Design review of the part shown in the three views and the two pictorial views. Dimensions are in mm from the part's minimum x, y and z. A direction names the side the tool comes from. Coordinates: 2 decimals unless noted, no trailing zeros. Order: outer loops, then holes, each group sorted by start corner. A loop starts at its lowest first (then second) coordinate and runs counter-clockwise, first axis right, second up. Notation, with made-up numbers: M 13,84 L 36,84 A10 ccw 36,95 Z; hole C -16.75,42 d11. An arc over 180 degrees is marked long. Use CSV: the item, a comma, the result in double quotes.
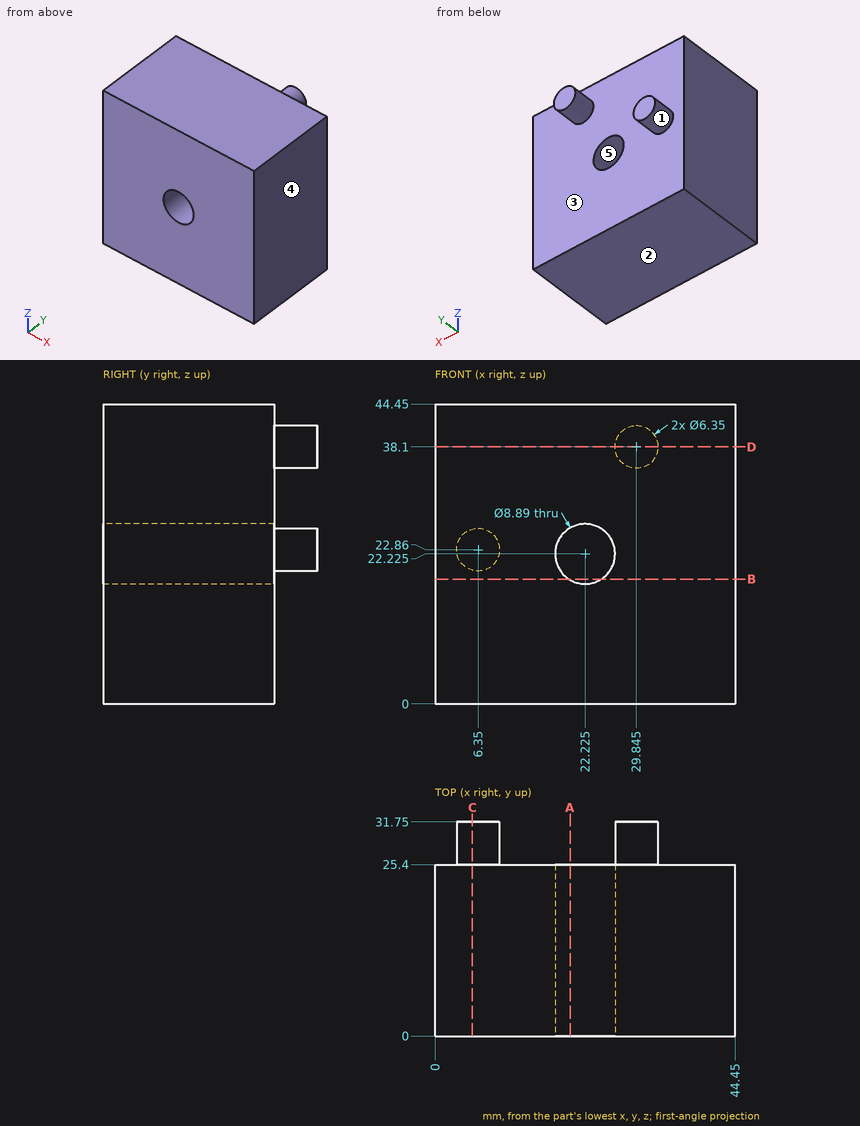
(1) For the marked faces 1 and 2, list the 3-axis set-ups (+Z, -Z, +X, -X, +Y, -Y) from which the entire face can be reached by the end or side of a thin tool; tool diameter is ignored.
The answers:
face 1,"+Y"
face 2,"-Z, +X, -X, +Y, -Y"
(2) The part is to be moulded in two halves that separate along X. For the marked faces 3, 4 and 5, say which applies: pulls with the +X half, pulls with the -X half, needs draft (parallel to the pull), parting line crosses it, or undercut.
The answers:
face 3,"needs draft"
face 4,"pulls with the +X half"
face 5,"undercut"
(3) Clearance check with a flat-ended pin moving along its axis: P1, Ø1, axis at x = 15, z = 11.5, coming from the +Y side. State where the tip first meets the part, or that it passes through.
The answers:
P1,"stops at y = 25.4"
(4) Add section C-C on x = 5.5. State the section outline as (y, z) points, and give its area (3 significant figures).
The answers:
outline,"M 0,0 L 25.4,0 L 25.4,19.8 L 31.75,19.8 L 31.75,25.92 L 25.4,25.92 L 25.4,44.45 L 0,44.45 Z"
area,"1,170 mm2"
(5) Wall thickness on probe 1 along Y at (x, z) = (12.5, 12); probe 2 along Z at (x, y) = (19.5, 8.5); probe 3 along Z at (x, y) = (23, 21): over which ranges is each line inside the solid? List them lowest first.
The answers:
probe 1,"y = 0 to 25.4"
probe 2,"z = 0 to 18.71, 25.74 to 44.45"
probe 3,"z = 0 to 17.85, 26.6 to 44.45"
(6) Add section A-A on x = 20. State the section outline as (y, z) points.
The answers:
outline,"M 0,0 L 25.4,0 L 25.4,18.38 L 0,18.38 Z; M 0,26.07 L 25.4,26.07 L 25.4,44.45 L 0,44.45 Z"
(7) Add section B-B on z = 18.5. State the section outline as (x, y) points.
The answers:
outline,"M 0,0 L 19.8,0 L 19.8,25.4 L 0,25.4 Z; M 24.65,0 L 44.45,0 L 44.45,25.4 L 24.65,25.4 Z"
(8) Add section D-D on z = 38.1. State the section outline as (x, y) points, and give its area (3 significant figures).
The answers:
outline,"M 0,0 L 44.45,0 L 44.45,25.4 L 33.02,25.4 L 33.02,31.75 L 26.67,31.75 L 26.67,25.4 L 0,25.4 Z"
area,"1,170 mm2"
